from build123d import *

# Parameters (mm, degrees)
ESQUISSE1_W              = 20
ESQUISSE1_H              = 17
ESQUISSE1_R              = 2.1
BOSS_EXTRU_1_DEPTH       = 5
ESQUISSE2_W              = 18
ESQUISSE2_H              = 4.4
BOSS_EXTRU_3_DEPTH       = 10
ESQUISSE5_W              = 6.5
ESQUISSE5_H              = 17
ENL_V_MAT_EXTRU_3_DEPTH  = 18
BOSS_EXTRU_6_DEPTH       = 8.4
BOSS_EXTRU_6_DEPTH_BACK  = 10
ESQUISSE10_W             = 7
ESQUISSE10_H             = 10
ESQUISSE11_W             = 5.5
ESQUISSE11_H             = 2.5
ESQUISSE11_W_2           = 7
ESQUISSE11_H_2           = 0.5
BOSS_EXTRU_7_DEPTH       = 17
ESQUISSE12_W             = 18
ESQUISSE12_H             = 2.5
BOSS_EXTRU_8_DEPTH       = 10
ESQUISSE20_R             = 2.25
ENL_V_MAT_EXTRU_7_DEPTH  = 18
ESQUISSE21_W             = 4
ESQUISSE21_H             = 10
ESQUISSE21_W_2           = 6.9
BOSS_EXTRU_9_DEPTH       = 25
ESQUISSE22_W             = 19.5
ESQUISSE22_H             = 10
BOSS_EXTRU_10_DEPTH      = 14
BOSS_EXTRU_11_DEPTH      = 3
CHANFREIN1_SIZE          = 1
ESQUISSE29_R             = 2.5
ENL_V_MAT_EXTRU_11_DEPTH = 10
ENL_V_START              = -7.5
ESQUISSE30_R             = 4.75
ESQUISSE30_R_2           = 2.5
ENL_V_MAT_EXTRU_12_DEPTH = 5.5


with BuildPart() as part:
    # Esquisse1 → Boss.-Extru.1 (new body)
    with BuildSketch(Plane.XY):
        with Locations((10, 8.5)):
            Rectangle(ESQUISSE1_W, ESQUISSE1_H)
        with Locations((10, 5)):
            Circle(ESQUISSE1_R, mode=Mode.SUBTRACT)
        with Locations((10, 12)):
            Circle(ESQUISSE1_R, mode=Mode.SUBTRACT)
    extrude(amount=BOSS_EXTRU_1_DEPTH)

    # Esquisse5 → Enlèv. mat.-Extru.3 (cut)
    with BuildSketch(Plane.XY.offset(5)):
        with Locations((16.75, 8.5)):
            Rectangle(ESQUISSE5_W, ESQUISSE5_H)
        with Locations((3.25, 8.5)):
            Rectangle(ESQUISSE5_W, ESQUISSE5_H)
    extrude(amount=-ENL_V_MAT_EXTRU_3_DEPTH, mode=Mode.SUBTRACT)



with BuildPart() as body_2:
    # Esquisse2 → Boss.-Extru.3 (new body)
    with BuildSketch(Plane.XZ):
        with Locations((10, -2.8)):
            Rectangle(ESQUISSE2_W, ESQUISSE2_H)
    extrude(amount=BOSS_EXTRU_3_DEPTH)


with BuildPart() as part_1:
    add(part.part)

    add(body_2.part)  # Boss.-Extru.6 merges body 2
    # Esquisse10 → Boss.-Extru.6 (add, two sides: drawn at the far end of the back side and taken through both)
    with BuildSketch(Plane.XY.offset(5).offset(-BOSS_EXTRU_6_DEPTH_BACK)):
        with Locations((10, -5)):
            Rectangle(ESQUISSE10_W, ESQUISSE10_H)
    extrude(amount=BOSS_EXTRU_6_DEPTH + BOSS_EXTRU_6_DEPTH_BACK)

    # Esquisse11 → Boss.-Extru.7 (add)
    with BuildSketch(Plane(origin=(0, 0, 0), x_dir=(1, 0, 0), z_dir=(0, 1, 0))):
        with Locations((3.75, 6.25)):
            Rectangle(ESQUISSE11_W, ESQUISSE11_H)
        with Locations((10, 6.25)):
            Rectangle(ESQUISSE11_W_2, ESQUISSE11_H)
        with Locations((16.25, 6.25)):
            Rectangle(ESQUISSE11_W, ESQUISSE11_H)
        with Locations((3.75, 4.75)):
            Rectangle(ESQUISSE11_W, ESQUISSE11_H_2)
        with Locations((10, 4.75)):
            Rectangle(ESQUISSE11_W_2, ESQUISSE11_H_2)
        with Locations((16.25, 4.75)):
            Rectangle(ESQUISSE11_W, ESQUISSE11_H_2)
    extrude(amount=BOSS_EXTRU_7_DEPTH)

    # Esquisse12 → Boss.-Extru.8 (add)
    with BuildSketch(Plane.XZ):
        with Locations((10, -6.25)):
            Rectangle(ESQUISSE12_W, ESQUISSE12_H)
    extrude(amount=BOSS_EXTRU_8_DEPTH)

    # Esquisse20 → Enlèv. mat.-Extru.7 (cut)
    with BuildSketch(Plane.XY.offset(5)):
        with Locations((10, 5)):
            Circle(ESQUISSE20_R)
        with Locations((10, 12)):
            Circle(ESQUISSE20_R)
    extrude(amount=-ENL_V_MAT_EXTRU_7_DEPTH, mode=Mode.SUBTRACT)

    # Esquisse21 → Boss.-Extru.9 (add)
    with BuildSketch(Plane(origin=(13.5, 0, 0), x_dir=(0, 0, -1), z_dir=(1, 0, 0))):
        with Locations((-11.4, -5)):
            Rectangle(ESQUISSE21_W, ESQUISSE21_H)
        with Locations((4.05, -5)):
            Rectangle(ESQUISSE21_W_2, ESQUISSE21_H)
    boss_extru_9 = extrude(amount=BOSS_EXTRU_9_DEPTH)

    # Esquisse22 → Boss.-Extru.10 (add)
    with BuildSketch(Plane.XY.offset(-0.6)):
        with Locations((28.75, -5)):
            Rectangle(ESQUISSE22_W, ESQUISSE22_H)
    boss_extru_10 = extrude(amount=BOSS_EXTRU_10_DEPTH)

    # Esquisse24 → Boss.-Extru.11 (add)
    with BuildSketch(Plane(origin=(0, 0, -7.5), x_dir=(-1, 0, 0), z_dir=(0, 0, -1))):
        Polygon((-38.5, 0), (-19, 0), (-19, 17), align=None)
    boss_extru_11 = extrude(amount=-BOSS_EXTRU_11_DEPTH)

    # Symétrie1: Boss.-Extru.9, Boss.-Extru.10, Boss.-Extru.11 across plane
    add(boss_extru_9.mirror(Plane.ZY.offset(-10)))
    add(boss_extru_10.mirror(Plane.ZY.offset(-10)))
    add(boss_extru_11.mirror(Plane.ZY.offset(-10)))

    # Chanfrein1
    chanfrein1_edges = [part_1.edges().sort_by_distance(p)[0] for p in [
        (10, 0, 5),
    ]]
    chamfer(chanfrein1_edges, length=CHANFREIN1_SIZE)

    # Esquisse29 → Enlèv. mat.-Extru.11 (cut)
    with BuildSketch(Plane(origin=(0, 0, 0), x_dir=(1, 0, 0), z_dir=(0, 1, 0))):
        with Locations(Location((-13.5, -4.4, 0), (0, 0, 270))):
            Circle(ESQUISSE29_R)
        with Locations(Location((33.5, -4.4, 0), (0, 0, 270))):
            Circle(ESQUISSE29_R)
    extrude(amount=-ENL_V_MAT_EXTRU_11_DEPTH, mode=Mode.SUBTRACT)

    # Esquisse30 → Enlèv. mat.-Extru.12 (cut)
    # profile 1 of 2: a face of its own
    with BuildSketch(Plane(origin=(0, -10, 0), x_dir=(-1, 0, 0), z_dir=(0, -1, 0)).offset(ENL_V_START)):
        with Locations((13.5, -4.4)):
            Circle(ESQUISSE30_R)
        with Locations(Location((13.5, -4.4, 0), (0, 0, 270))):
            Circle(ESQUISSE30_R_2, mode=Mode.SUBTRACT)
    # profile 2 of 2: a face of its own
    with BuildSketch(Plane(origin=(0, -10, 0), x_dir=(-1, 0, 0), z_dir=(0, -1, 0)).offset(ENL_V_START)):
        with BuildLine():
            ThreePointArc((18.25, -4.4), (16.858757211, -7.758757211), (13.5, -9.15))
            Line((13.5, -9.15), (18.5, -9.15))
            Line((18.5, -9.15), (18.5, 0.35))
            Line((18.5, 0.35), (13.5, 0.35))
            ThreePointArc((13.5, 0.35), (16.858757211, -1.041242789), (18.25, -4.4))
        make_face()
    enl_v_mat_extru_12 = extrude(amount=ENL_V_MAT_EXTRU_12_DEPTH, mode=Mode.SUBTRACT)

    # Symétrie3: Enlèv. mat.-Extru.12 across plane
    add(enl_v_mat_extru_12.mirror(Plane.ZY.offset(-10)), mode=Mode.SUBTRACT)


solid = part_1.part
Geometry: final body of the model. Coordinates: model frame, mm. A direction names the side the tool comes from. Give positions to 0.01 mm unless a question says otherwise; leave off trailing zeros. Write each loop counter-clockwise with the first axis right and the second up, starting at its lowest first coordinate (ties: lowest second). Pieces come first, ordered by that corner, then holes. Notation, with made-up numbers: M 72,24 L 84,24 A16 ccw 84,37 Z; hole C 36,55 d1. An arc over 180 degrees is marked long. Answer in a Markdown table with one row per item. Add a question column.
(1) Section A-A on x = 10. Return loops of the section in (y, z).
(2) Section B-B on z = 4.4. State how many separate pieces and enclosed holes the cut face has, and give its area (3 significant figures).
(3) Ray query, line 1 (Y direction, x = 10, z = -6.05); line 2 (X direction, y = -8.75, z = 4.4); line 3 (Z direction, x = 36, y = -4). Return the intervals inside material, ascending.
(4) Section D-D on z = -5.75. Return loops of the section in (x, y), and give its area (3 significant figures).
(5) Mould query, pull axis X, two halves, no side actions, for faces 1 (the flat face through (-18.5, -2, 3)), 2 (the flat face through (10, 17, -6)), 3 (the flat face through (16, -5, 9.4)). Classes: +X half, -X half, draft (parallel to the pull), parting line (faces both ways), or undercut.
(6) Section C-C on y = 5. Return loops of the section in (x, z), and give its area (3 significant figures).
(7) Reachability of faces 4 (the flat face through (4, -5, 9.4)), 5 (the flat face through (28.61, 8.62, -6.02)), 6 (the flat face through (-8.61, 8.62, -6.02)), 7 (the cylindrical face through (28.75, -5.21, 4.3)), 8 (the flat face through (-16, -5, -0.35)) from +Z, -Z, +X, -X, +Y, -Y: full face, straight path, thin tool, end or side. Return the list, or none.
(8) First-contact query: pin 1 (3.5 mm diameter, centred on x = 10, y = 12, fed in from -Z); pin 2 (10.5 mm diameter, centred on x = -12, z = 6, fed in from +Y); pin 3 (4 mm diameter, centred on x = 32.5, y = 4, fed in from +Z); pin 4 (1.5 mm diameter, centred on y = 1, z = 6, fed in from -X). Flat tips, straight axial feed; report the tip coordinate or a pass-through.
Result set:
| question | item | result |
|---|---|---|
| 1 | outline | M -10,-7.5 L 2.75,-7.5 L 2.75,-4.5 L 0,-4.5 L 0,0 L 2.75,0 L 2.75,5 L 1,5 L 0,6 L 0,13.4 L -10,13.4 Z; M 7.25,-7.5 L 9.75,-7.5 L 9.75,-4.5 L 7.25,-4.5 Z; M 7.25,0 L 9.75,0 L 9.75,5 L 7.25,5 Z; M 14.25,-7.5 L 17,-7.5 L 17,-4.5 L 14.25,-4.5 Z; M 14.25,0 L 17,0 L 17,5 L 14.25,5 Z |
| 2 | separate pieces | 7 |
| 2 | enclosed holes | 2 |
| 2 | area | 395 mm^2 |
| 3 | line 1 | y = -10 to 2.75, 7.25 to 9.75, 14.25 to 17 |
| 3 | line 2 | x = -18.5 to -16, -11 to 1, 6.5 to 13.5, 19 to 31, 36 to 38.5 |
| 3 | line 3 | z = -7.5 to -0.35, 9.15 to 13.4 |
| 4 | outline | M -18.5,-10 L 38.5,-10 L 38.5,0 L 19,17 L 1,17 L -18.5,0 Z; hole C 10,5 d4.5; hole C 10,12 d4.5 |
| 4 | area | 1,180 mm^2 |
| 5 | face 1 | -X half |
| 5 | face 2 | draft |
| 5 | face 3 | undercut |
| 6 | outline | M -12.76,-7.5 L 7.75,-7.5 L 7.75,-4.5 L -12.76,-4.5 Z; M 6.5,0 L 7.75,0 L 7.75,5 L 6.5,5 Z; M 12.25,-7.5 L 32.76,-7.5 L 32.76,-4.5 L 12.25,-4.5 Z; M 12.25,0 L 13.5,0 L 13.5,5 L 12.25,5 Z |
| 6 | area | 136 mm^2 |
| 7 | face 4 | +Y, -Y |
| 7 | face 5 | +Z, -Z, +X, +Y |
| 7 | face 6 | +Z, -Z, -X, +Y |
| 7 | face 7 | +X |
| 7 | face 8 | -X |
| 8 | pin 1 | passes through |
| 8 | pin 2 | stops at y = 0 |
| 8 | pin 3 | stops at z = -4.5 |
| 8 | pin 4 | stops at x = 6.5 |
